```python
from build123d import *

# Parameters (mm, degrees)
POCKET_DEPTH = 2


with BuildPart() as part:
    # Sketch → Revolution (revolve)
    with BuildSketch(Plane.YZ):
        Polygon((-3.5, 4), (-3.5, 0), (0, 0), (0, 34), (-2, 34), (-2, 4), align=None)
    revolve(axis=Axis((0, 0, 0), (0, 0, 1)))

    # Sketch001 (on Face2 of Revolution) → Pocket (cut)
    with BuildSketch(Plane.YX):
        Polygon((0, 2.5), (-2.165064, 1.25), (-2.165064, -1.25), (0, -2.5), (2.165064, -1.25), (2.165064, 1.25), align=None)
    extrude(amount=-POCKET_DEPTH, mode=Mode.SUBTRACT)


solid = part.part
```
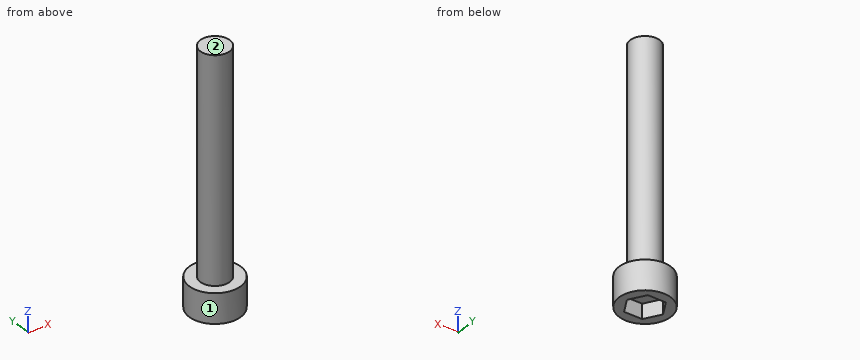
Source: CAD feature listing. Evaluate the final solid. Frame: model axes, mm. Face numbers are marked on the shaded views. Round coordinates to 2 decimals unless told otherwise and drop trailing zeros. Write each loop counter-clockwise with the first axis right and the second up, starting at its lowest first coordinate (ties: lowest second). Pieces come first, ordered by that corner, then holes. Notation, with made-up numbers: M -24.75,84.5 L -13.75,84.5 A28 cw -13.75,105.5 Z; hole C 77,-3 d6. An arc over 180 degrees is marked long. Use CSV: the item, a comma, the result in double quotes. Start each with the question number.
Q1. Line query: line 1 (Z direction, x = -1.5, y = 0.75); line 2 (Z direction, x = 2, y = -2); line 3 (X direction, y = 0.75, z = 15.5). Output: solid intervals per line, ascending. Write a range as from..to.
Q2. Cut plane D-D on y = 2.75. Output: boundary loops of the cut face in (x, z), plus the area to 3 significant figures.
Q3. Cut plane A-A on x = 0. Output: boundary loops of the cut face in (y, z).
Q4. Cut plane B-B on y = 0.5. Output: boundary loops of the cut face in (x, z).
Q5. Cut plane C-C on z = 16. Output: boundary loops of the cut face in (x, y).
Q6. First-contact query: P1, Ø3.5, axis at x = 0, y = 0, coming from the -Z side. Flat tip, straight axial feed; report the tip coordinate or a pass-through.
Q7. Pull-direction query (Y, two-part tool) for the marked faces 1 and 2; classes: +Y half, -Y half, draft (parallel to the pull), parting line (faces both ways), or undercut.
Results found:
1,line 1,"2..34"
1,line 2,"0..4"
1,line 3,"-1.85..1.85"
2,outline,"M -2.17,0 L 2.17,0 L 2.17,4 L -2.17,4 Z"
2,area,"17.3 mm^2"
3,outline,"M -3.5,0 L -2.17,0 L -2.17,2 L 2.17,2 L 2.17,0 L 3.5,0 L 3.5,4 L 2,4 L 2,34 L -2,34 L -2,4 L -3.5,4 Z"
4,outline,"M -3.46,0 L -2.21,0 L -2.21,2 L 2.21,2 L 2.21,0 L 3.46,0 L 3.46,4 L 1.94,4 L 1.94,34 L -1.94,34 L -1.94,4 L -3.46,4 Z"
5,outline,"C 0,0 d4"
6,P1,"z = 2"
7,face 1,"parting line"
7,face 2,"draft"
